from build123d import *

# Parameters (mm, degrees)
PAD041_DEPTH        = 10
SKETCH094_R         = 15.975
POCKET017_DEPTH     = 5
SKETCH093_R         = 15
POCKET018_DEPTH     = 5
HOLE016_D           = 2.5
HOLE016_DEPTH       = 25
HOLE016_CSINK_D     = 6.1
HOLE016_CSINK_ANGLE = 90
SKETCH096_R         = 1.25
HOLE017_DEPTH       = 14.248924
HOLE017_TIPS_R      = 1.25
SKETCH097_R         = 1.25
HOLE018_DEPTH       = 14.248924
HOLE018_TIPS_R      = 1.25
SKETCH_R            = 1.25
HOLE_DEPTH          = 14.248924
HOLE_TIPS_R         = 1.25


with BuildPart() as part:
    # Sketch092 → Pad041 (new body)
    with BuildSketch(Plane.XY):
        Polygon((86.60254, 50), (0, 100), (-86.60254, 50), (-86.60254, -50), (0, -100), (86.60254, -50), align=None)
    extrude(amount=PAD041_DEPTH)

    # Sketch094 → Pocket017 (cut)
    with BuildSketch(Plane(origin=(0, 0, 0), x_dir=(1, 0, 0), z_dir=(0, 0, -1))):
        Circle(SKETCH094_R)
    extrude(amount=-POCKET017_DEPTH, mode=Mode.SUBTRACT)

    # Sketch093 → Pocket018 (cut)
    with BuildSketch(Plane.XY.offset(10)):
        Circle(SKETCH093_R)
    extrude(amount=-POCKET018_DEPTH, mode=Mode.SUBTRACT)

    # Hole016
    with Locations(Plane.XY.offset(10)):
        with Locations((0, 40.414519), (35, -20.207259), (-35, -20.207259)):
            CounterSinkHole(HOLE016_D / 2, HOLE016_CSINK_D / 2, depth=HOLE016_DEPTH, counter_sink_angle=HOLE016_CSINK_ANGLE)

    # Sketch096 (on Face2 of Hole016) → Hole017 (cut)
    with BuildSketch(Plane.YZ.offset(86.60254)):
        with Locations((0, 5)):
            Circle(SKETCH096_R)
    extrude(amount=-HOLE017_DEPTH, mode=Mode.SUBTRACT)

    # Hole017 tips → Hole017 tip 1 section 0
    with BuildSketch(Plane.YZ.offset(72.353616), mode=Mode.PRIVATE) as hole017_tip_1_s0:
        with Locations((0, 5)):
            Circle(HOLE017_TIPS_R)
    loft([hole017_tip_1_s0.sketch, Vertex(71.60254, 0, 5)], mode=Mode.SUBTRACT)

    # Sketch097 (on Face3 of Hole017) → Hole018 (cut)
    with BuildSketch(Plane(origin=(-43.30127, 75, 0), x_dir=(-0.866025, -0.5, 0), z_dir=(-0.5, 0.866025, 0))):
        with Locations((0, 5)):
            Circle(SKETCH097_R)
    extrude(amount=-HOLE018_DEPTH, mode=Mode.SUBTRACT)

    # Hole018 tips → Hole018 tip 1 section 0
    with BuildSketch(Plane(origin=(-36.176808, 62.66007, 0), x_dir=(-0.866025, -0.5, 0), z_dir=(-0.5, 0.866025, 0)), mode=Mode.PRIVATE) as hole018_tip_1_s0:
        with Locations((0, 5)):
            Circle(HOLE018_TIPS_R)
    loft([hole018_tip_1_s0.sketch, Vertex(-35.80127, 62.009619, 5)], mode=Mode.SUBTRACT)

    # Sketch (on Face10 of Hole018) → Hole (cut)
    with BuildSketch(Plane(origin=(-43.30127, -75, 0), x_dir=(0.866025, -0.5, 0), z_dir=(-0.5, -0.866025, 0))):
        with Locations((0, 5)):
            Circle(SKETCH_R)
    extrude(amount=-HOLE_DEPTH, mode=Mode.SUBTRACT)

    # Hole tips → Hole tip 1 section 0
    with BuildSketch(Plane(origin=(-36.176808, -62.66007, 0), x_dir=(0.866025, -0.5, 0), z_dir=(-0.5, -0.866025, 0)), mode=Mode.PRIVATE) as hole_tip_1_s0:
        with Locations((0, 5)):
            Circle(HOLE_TIPS_R)
    loft([hole_tip_1_s0.sketch, Vertex(-35.80127, -62.009619, 5)], mode=Mode.SUBTRACT)


solid = part.part
Here's how the part is built. I have some questions about the finished solid (model axes, mm). Give positions to 0.01 mm unless a question says otherwise; leave off trailing zeros. Order: outer loops, then holes, each group sorted by start corner. A loop starts at its lowest first (then second) coordinate and runs counter-clockwise, first axis right, second up. Notation, with made-up numbers: (-34.5, -4.75) -> (-20.5, -4.75) arc R29 cw to (-20.5, 25.25) -> close; hole circle Ø3 at (28, 38). An arc over 180 degrees is marked (long way). One line per item, written item: value. Start each with the question number.
1. Will these pins go through, and if not, where does the flat tip stop? pin 1 Ø1.5 at (x, z) = (54, 9) entering from +Y; pin 2 Ø2 at (y, z) = (-54, 4) entering from -X; pin 3 Ø1.5 at (y, z) = (0, 5) entering from +X.
2. Imagine slicing it at B-B, the plane x = -20.5. List the corners of the cut face in (y, z) for me.
3. Imagine slicing it at A-A, the plane y = 58.5. List the corners of the cut face in (x, z) for me.
4. We'd pull the mould along X, two halves only. Please class faces 1 (the face through (-40.29, 68.63, 3.89)), 2 (the face through (-42.695, 75.35, 7.152)), 3 (the face through (-3.463, 15.595, 2.465)), 4 (the face through (86.603, -1, 6)): released by +X, released by -X, zero draft, split by the parting line, or undercut.
5. I need wall thicknesses on probe 1 along Y at (x, z) = (0, 6.75); probe 2 along Y at (x, z) = (0, 2.5) (3 decimals); probe 3 along Z at (x, y) = (81, 0). Which ranges of each line are inside material? Lowest first, please. Write a range as from..to.
Values follow:
1. pin 1: stops at y = 69.26
1. pin 2: stops at x = -81.41
1. pin 3: stops at x = 72.05
2. outline: (-88.16, 0) -> (88.16, 0) -> (88.16, 10) -> (-88.16, 10) -> close
3. outline: (-71.88, 0) -> (71.88, 0) -> (71.88, 10) -> (-71.88, 10) -> close
4. face 1: undercut
4. face 2: released by -X
4. face 3: undercut
4. face 4: released by +X
5. probe 1: y = -100..-15, 15..39.16, 41.66..100
5. probe 2: y = -100..-15.975, 15.975..39.165, 41.665..100
5. probe 3: z = 0..3.75, 6.25..10
